Build history of the part. All positions in model axes, mm. Give positions to 0.01 mm unless a question says otherwise; leave off trailing zeros. Write each loop counter-clockwise with the first axis right and the second up, starting at its lowest first coordinate (ties: lowest second). Pieces come first, ordered by that corner, then holes. Notation, with made-up numbers: M -7.75,-16 L 20.25,-16 A12 cw 20.25,0 Z; hole C 78.5,60 d4. An arc over 180 degrees is marked long. Return JSON: item names as keys, results as strings. Group by question number.
Q1. Wall check: probe 1 along Y at (x, z) = (8.5, 0.25); probe 2 along Y at (x, z) = (-5.5, 0.4); probe 3 along X at (y, z) = (15.75, 0.15). Give the ranges that are in metal, low to high.
Q2. Band-saw the part on B-B, the plane x = 3. Give the cut face in (y, z), then the cut area to 3 significant figures.
Q3. Band-saw the part on D-D, the plane z = 0.4. Count the separate pieces of the cut face and the enclosed holes in it, then the cut area to 3 significant figures.
Q4. Band-saw the part on A-A, the plane y = 23. Give the cut face in (x, z).
Q5. Band-saw the part on C-C, the plane x = -7.5. Give the cut face in (y, z).
Q6. Flat gauge pin, fed straight in: pin 1 Ø5.5 at (x, y) = (-6.58, 19.71) entering from -Z. Where does the tip first touch, or does it go through?
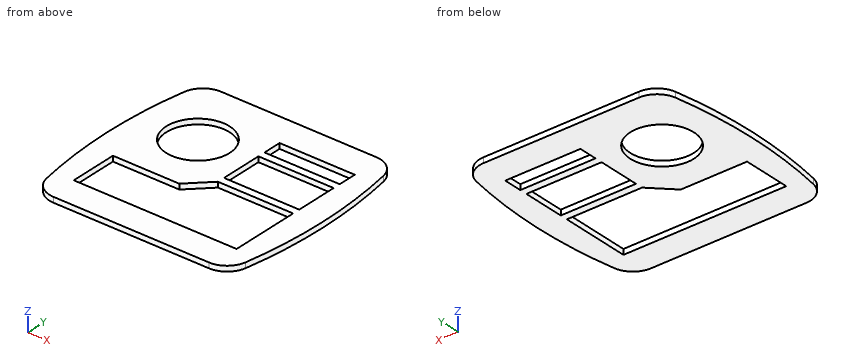
from build123d import *

# Parameters (mm, degrees)
F0_R     = 4.5466
F0_W     = 10.795
F0_H     = 6.0198
F0_H_2   = 2.6416
F1_DEPTH = 0.762


with BuildPart() as f1:
    # F0 (on Top) → F1 (new body)
    with BuildSketch(Plane.XY):
        with BuildLine():
            ThreePointArc((-14.2875, 2.604771), (-13.197614, 0.73665), (-11.164126, 0))
            Line((-11.164126, 0), (11.164126, 0))
            ThreePointArc((11.164126, 0), (13.197614, 0.73665), (14.2875, 2.604771))
            ThreePointArc((14.2875, 2.604771), (15.3797, 14.6685), (14.2875, 26.732229))
            ThreePointArc((14.2875, 26.732229), (13.197614, 28.60035), (11.164126, 29.337))
            Line((11.164126, 29.337), (-11.164126, 29.337))
            ThreePointArc((-11.164126, 29.337), (-13.197614, 28.60035), (-14.2875, 26.732229))
            ThreePointArc((-14.2875, 26.732229), (-15.3797, 14.6685), (-14.2875, 2.604771))
        make_face()
        Polygon((0.889, 14.097), (11.684, 14.097), (11.684, 4.191), (-11.684, 4.191), (-11.684, 11.049), (-2.159, 11.049), align=None, mode=Mode.SUBTRACT)
        with Locations((-6.579606, 19.7104)):
            Circle(F0_R, mode=Mode.SUBTRACT)
        with Locations((6.2865, 18.1737)):
            Rectangle(F0_W, F0_H, mode=Mode.SUBTRACT)
        with Locations((6.2865, 23.5712)):
            Rectangle(F0_W, F0_H_2, mode=Mode.SUBTRACT)
    extrude(amount=F1_DEPTH)


solid = f1.part
From the geometry:
{
 "1": {"probe 1": "y = 0 to 4.19, 14.1 to 15.16, 21.18 to 22.25, 24.89 to 29.34", "probe 2": "y = 0 to 4.19, 11.05 to 15.29, 24.13 to 29.34", "probe 3": "x = -15.37 to -8.81, -4.35 to 0.89, 11.68 to 15.37"},
 "2": {"outline": "M 0,0 L 4.19,0 L 4.19,0.76 L 0,0.76 Z; M 14.1,0 L 15.16,0 L 15.16,0.76 L 14.1,0.76 Z; M 21.18,0 L 22.25,0 L 22.25,0.76 L 21.18,0.76 Z; M 24.89,0 L 29.34,0 L 29.34,0.76 L 24.89,0.76 Z", "area": "8.21 mm^2"},
 "3": {"separate pieces": "1", "enclosed holes": "4", "area": "509 mm^2"},
 "4": {"outline": "M -14.86,0 L -9.72,0 L -9.72,0.76 L -14.86,0.76 Z; M -3.44,0 L 0.89,0 L 0.89,0.76 L -3.44,0.76 Z; M 11.68,0 L 14.86,0 L 14.86,0.76 L 11.68,0.76 Z"},
 "5": {"outline": "M 0,0 L 4.19,0 L 4.19,0.76 L 0,0.76 Z; M 11.05,0 L 15.26,0 L 15.26,0.76 L 11.05,0.76 Z; M 24.16,0 L 29.34,0 L 29.34,0.76 L 24.16,0.76 Z"},
 "6": {"pin 1": "passes through"}
}
